Check sheet for the drawn part. Datum: minimum x, y, z corner. Units: mm. A direction names the side the tool comes from. Give positions to 0.01 mm unless a question says otherwise; leave off trailing zeros. Order: outer loops, then holes, each group sorted by start corner. A loop starts at its lowest first (then second) coordinate and runs counter-clockwise, first axis right, second up. Notation, with made-up numbers: M 27.25,80 L 55.25,80 A11 ccw 55.25,99 Z; hole C 87.25,11.5 d5. An arc over 180 degrees is marked long. Put each result on its own line as item: value. Start each with the question number.
Q1. Material ranges on L1, parallel to Y at x = 1.2, z = 23.2; L2, parallel to Z at x = 1.75, y = 20; L3, parallel to Z at x = 4.1, y = 20.5, recorded low to high.
Q2. Section check C-C on x = 4.1. Record the cut outline in (y, z).
Q3. Go/stop test with flat-tipped pins: pin 1 (0.8 mm diameter, centred on x = 1.5, z = 48.5, fed in from -Y); pin 2 (2 mm diameter, centred on x = 4, y = 33, fed in from +Z); pin 3 (0.8 mm diameter, centred on x = 2.5, z = 48.5, fed in from +Y); pin 4 (0.8 mm diameter, centred on x = 3, z = 41, fed in from -Y). Record where each tip stops, or that it passes through.
Q4. Section check B-B on z = 23.2. Record the cut outline in (x, y), then the cut area to 3 significant figures.
Q5. Access from +Z, -Z, +X, -X, +Y, -Y to the whole of each face (thin tool, end or side, straight path). Record for the marked faces 1, 2, 3, 4 and 5.
Q6. Mould release check, pull along Y, two halves, no side actions. Record for the marked faces 6, 7 and 8: +Y half, -Y half, draft (parallel to the pull), parting line (faces both ways), or undercut.
Q7. Section check A-A on y = 20. Record the cut outline in (x, z).
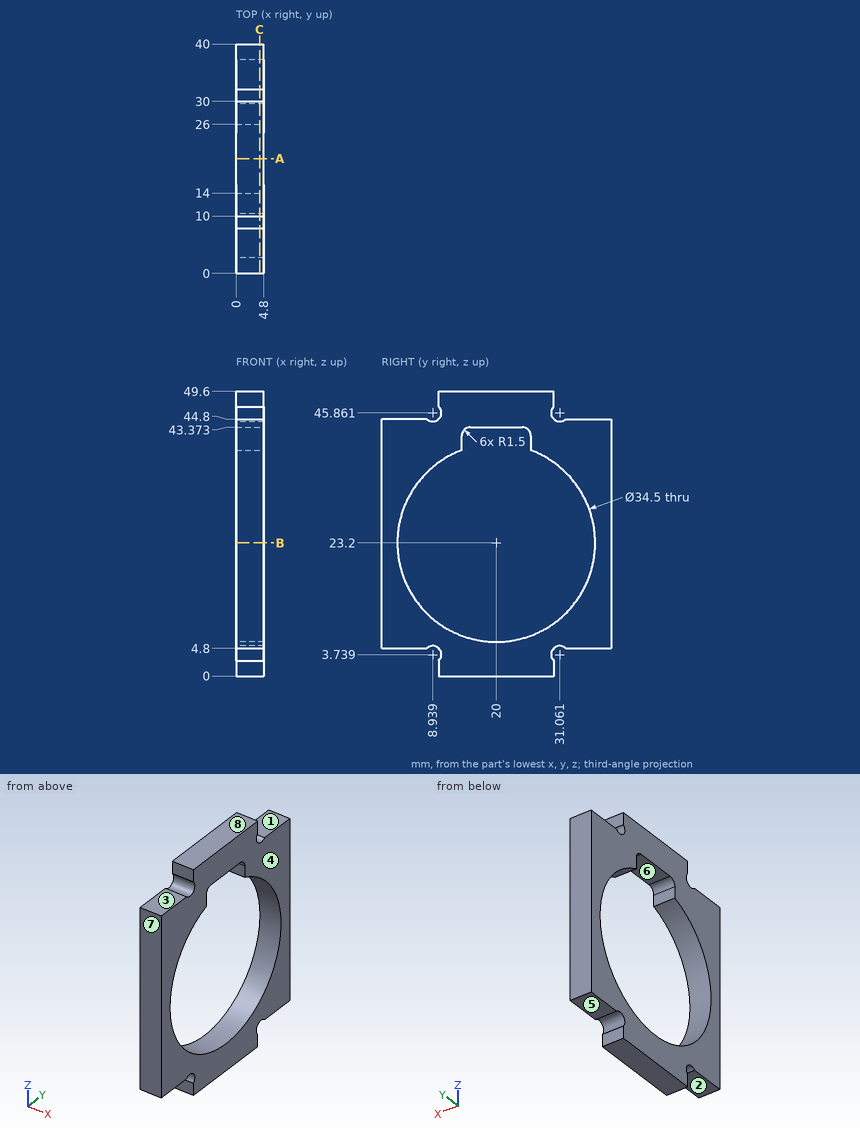
Results found:
1. L1: y = 0 to 2.75, 37.25 to 40
1. L2: z = 0 to 5.95, 43.37 to 49.6
1. L3: z = 0 to 5.96, 43.37 to 49.6
2. outline: M 0,4.8 L 7.88,4.8 A1.5 cw 10,2.68 L 10,0 L 30,0 L 30,2.68 A1.5 cw 32.12,4.8 L 40,4.8 L 40,44.8 L 32.12,44.8 A1.5 cw 30,46.92 L 30,49.6 L 10,49.6 L 10,46.92 A1.5 cw 7.88,44.8 L 0,44.8 Z; hole M 14,39.37 A17.25 ccw long 26,39.37 L 26,41.87 A1.5 ccw 24.5,43.37 L 15.5,43.37 A1.5 ccw 14,41.87 Z
3. pin 1: stops at y = 10
3. pin 2: stops at z = 44.8
3. pin 3: stops at y = 30
3. pin 4: stops at y = 0
4. outline: M 0,0 L 4.8,0 L 4.8,2.75 L 0,2.75 Z; M 0,37.25 L 4.8,37.25 L 4.8,40 L 0,40 Z
4. area: 26.4 mm^2
5. face 1: +Z, +X, -X, +Y
5. face 2: -Z, +X, -X, -Y
5. face 3: +Z, +X, -X, -Y
5. face 4: +Z, -Z, +X, +Y, -Y
5. face 5: -Z, +X, -X, +Y
6. face 6: undercut
6. face 7: -Y half
6. face 8: draft
7. outline: M 0,0 L 4.8,0 L 4.8,5.95 L 0,5.95 Z; M 0,43.37 L 4.8,43.37 L 4.8,49.6 L 0,49.6 Z
